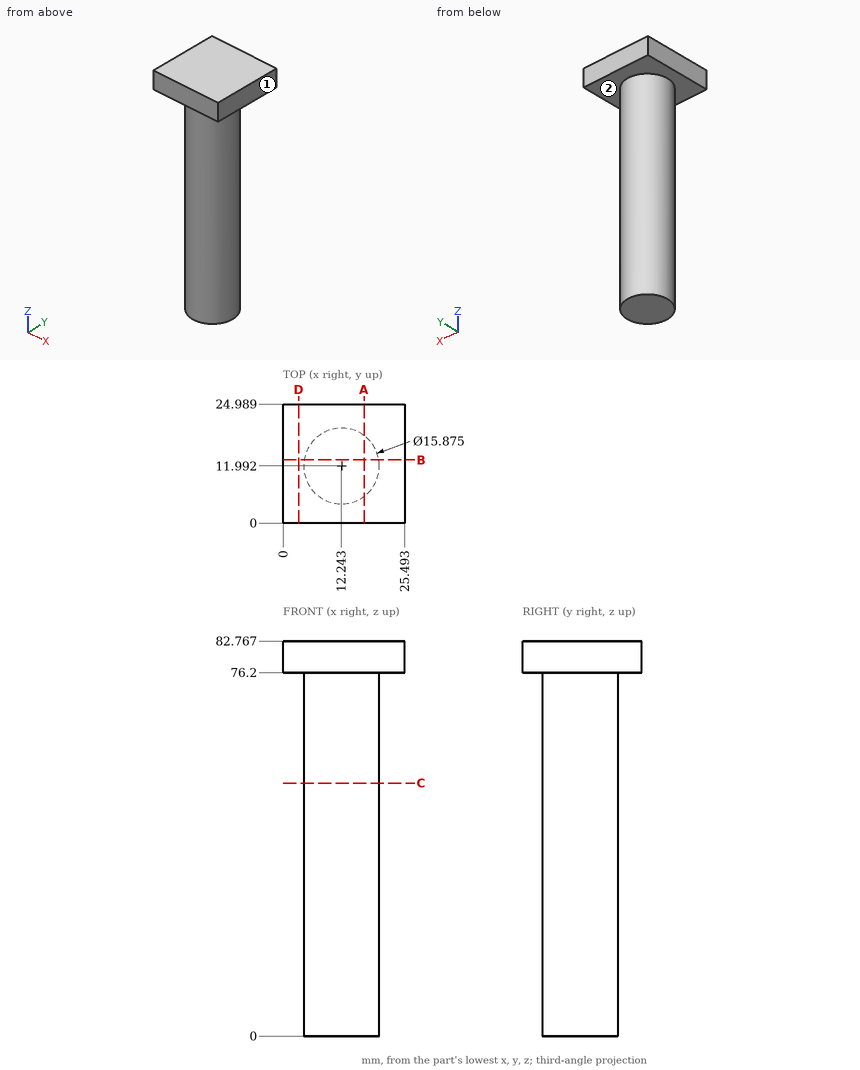
Answer from the drawing. Dimensions are ordinates in mm from the lowest x, y and z of the part. A direction names the side the tool comes from. Coordinates: 2 decimals unless noted, no trailing zeros. Write each loop counter-clockwise with the first axis right and the second up, starting at its lowest first coordinate (ties: lowest second). Pieces come first, ordered by that corner, then holes. Notation, with made-up numbers: (47, 71) - (103, 71) arc R20 ccw to (103, 110) - close; hole circle Ø5 at (-4.5, 87.5). An arc over 180 degrees is marked (long way). Answer as CSV lines item,"result".
1. Find section B-B (y = 13.25). Give the vertices of the cut face in (x, z), plus the area to 3 significant figures.
Computed values:
outline,"(0, 76.2) - (4.41, 76.2) - (4.41, 0) - (20.08, 0) - (20.08, 76.2) - (25.49, 76.2) - (25.49, 82.77) - (0, 82.77) - close"
area,"1,360 mm²"
2. Find section D-D (x = 3.25). Give the vertices of the cut face in (y, z), plus the area to 3 significant figures.
Computed values:
outline,"(0, 76.2) - (24.99, 76.2) - (24.99, 82.77) - (0, 82.77) - close"
area,"164 mm²"
3. Find section A-A (x = 17). Give the vertices of the cut face in (y, z) (1 decimal), plus the area to 3 significant figures.
Computed values:
outline,"(0, 76.2) - (5.6, 76.2) - (5.6, 0) - (18.3, 0) - (18.3, 76.2) - (25, 76.2) - (25, 82.8) - (0, 82.8) - close"
area,"1,130 mm²"
4. Given P1, Ø5, axis at x = 14, z = 23, coming from the +Y side; P2, Ø10, axis at x = 5.5, y = 7.5, coming from the -Z side; P3, Ø1, axis at y = 15, z = 37, coming from the +X side; P4, Ø1.5, axis at y = 13.5, z = 58.5, coming from the -X side, each flat-ended and moving along its own axis, determine where each tip first touches the part or whether it passes through.
Computed values:
P1,"stops at y = 19.93"
P2,"stops at z = 0"
P3,"stops at x = 19.77"
P4,"stops at x = 4.34"
5. Find section C-C (z = 53). Give the vertices of the cut face in (x, y) (1 decimal), plus the area to 3 significant figures.
Computed values:
outline,"circle Ø15.9 at (12.2, 12)"
area,"198 mm²"
6. A tool of negligible diameter and unlimited length cuts with its end or side. For the marked faces 1 and 2, from which of +Z, -Z, +X, -X, +Y, -Y can it reach the whole face along a straight path? Write none if from no direction.
Computed values:
face 1,"+Z, -Z, +X, +Y, -Y"
face 2,"-Z"
7. Straight lines are drawn through the part: line 1 (Z direction, x = 23, y = 5.75); line 2 (X direction, y = 12.25, z = 4.5); line 3 (X direction, y = 10.75, z = 58). For each, find the intervals that lie inside material, in ascending order. Write a range as [from, to].
Computed values:
line 1,"z = [76.2, 82.77]"
line 2,"x = [4.31, 20.18]"
line 3,"x = [4.4, 20.08]"
